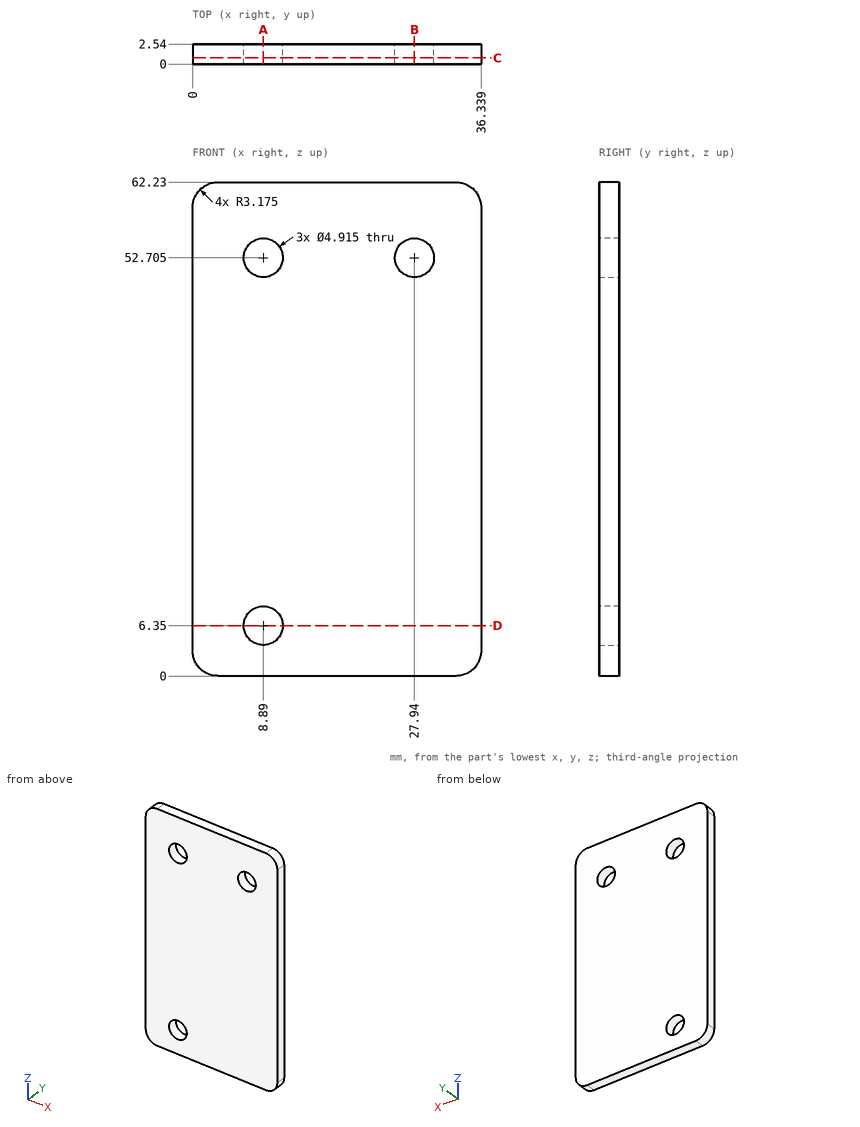
For this review, use the dimensioned drawing (mm, ordinates from the lowest corner) and the shaded views. Coordinates: 2 decimals unless noted, no trailing zeros. Loops run counter-clockwise (first coordinate to the right, second up) from the corner with the lowest first, then second, coordinate; pieces in that order, holes last. Notation, with made-up numbers: (41, -16.75) -> (60, -16.75) arc R12 ccw to (60, -9.75) -> close; hole circle Ø3 at (-27.75, -5). An arc over 180 degrees is marked (long way). Use a Markdown table: item, result. Add a question column.
Item 1: Clearance check with a flat-ended pin moving along its axis: P1, Ø3, axis at x = 8.89, z = 52.705, coming from the -Y side. State where the tip first meets the part, or that it passes through.
Item 2: We need section B-B, the plane x = 27.94. Write out the cut boundary in (y, z).
Item 3: We need section A-A, the plane x = 8.89. Write out the cut boundary in (y, z).
Item 4: We need section C-C, the plane y = 0.8. Count the separate pieces of the cut face and the enclosed holes in it, and give its area (3 significant figures).
Item 5: We need section D-D, the plane z = 6.35. Write out the cut boundary in (x, y).
Item 6: Wall thickness on L1, parallel to Z at x = 8.5, y = 1; L2, parallel to X at y = 2.05, z = 6.35; L3, parallel to Z at x = 30, y = 2.35 (1 decimal): over which ranges is each line inside the solid? List them lowest first. Write a range as from..to.
Numbers:
| question | item | result |
|---|---|---|
| 1 | P1 | passes through |
| 2 | outline | (0, 0) -> (2.54, 0) -> (2.54, 50.25) -> (0, 50.25) -> close; (0, 55.16) -> (2.54, 55.16) -> (2.54, 62.23) -> (0, 62.23) -> close |
| 3 | outline | (0, 0) -> (2.54, 0) -> (2.54, 3.89) -> (0, 3.89) -> close; (0, 8.81) -> (2.54, 8.81) -> (2.54, 50.25) -> (0, 50.25) -> close; (0, 55.16) -> (2.54, 55.16) -> (2.54, 62.23) -> (0, 62.23) -> close |
| 4 | separate pieces | 1 |
| 4 | enclosed holes | 3 |
| 4 | area | 2,200 mm^2 |
| 5 | outline | (0, 0) -> (6.43, 0) -> (6.43, 2.54) -> (0, 2.54) -> close; (11.35, 0) -> (36.34, 0) -> (36.34, 2.54) -> (11.35, 2.54) -> close |
| 6 | L1 | z = 0..3.92, 8.78..50.28, 55.13..62.23 |
| 6 | L2 | x = 0..6.43, 11.35..36.34 |
| 6 | L3 | z = 0..51.4, 54..62.2 |
